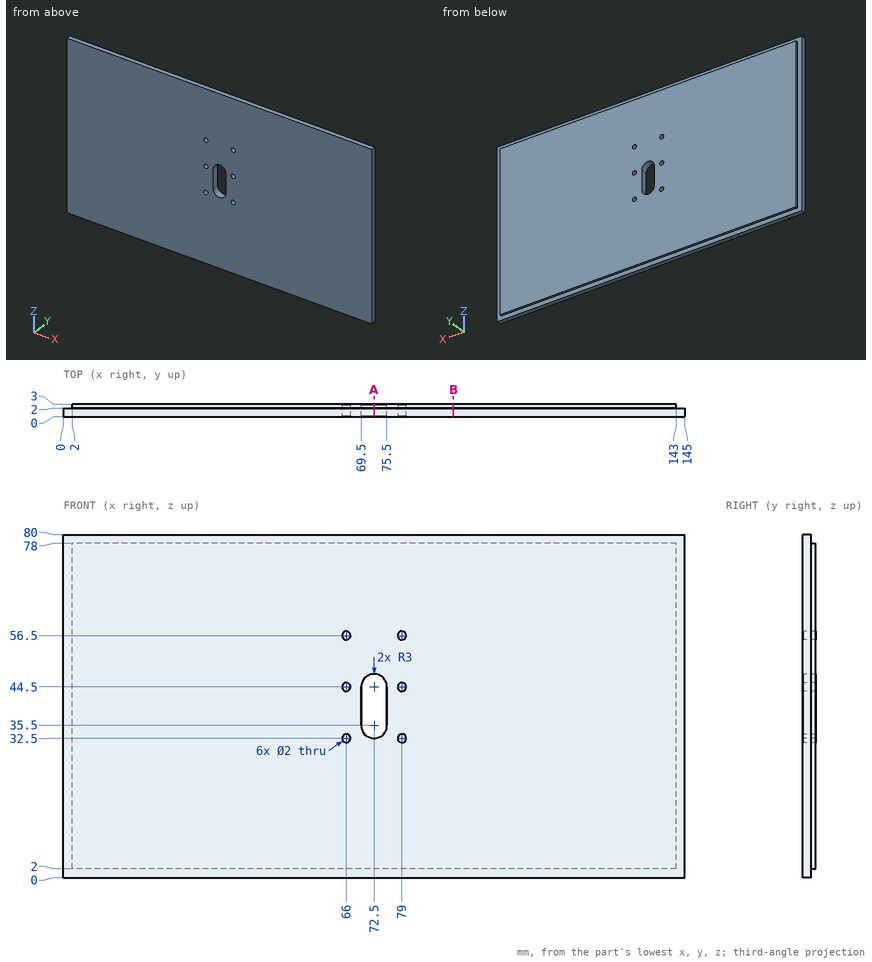
Check sheet for the drawn part. Datum: minimum x, y, z corner. Units: mm. Give positions to 0.01 mm unless a question says otherwise; leave off trailing zeros. Write each loop counter-clockwise with the first axis right and the second up, starting at its lowest first coordinate (ties: lowest second). Pieces come first, ordered by that corner, then holes. Notation, with made-up numbers: M 27.25,50.25 L 70.25,50.25 A30 ccw 70.25,83.25 Z; hole C 81.25,46.25 d8. An arc over 180 degrees is marked long. One line per question, with ' | ' between items.
1. Gauge pin test, flat ends, axial feed: pin 1 (1.2 mm diameter, centred on x = 66, z = 44.5, fed in from +Y); pin 2 (0.8 mm diameter, centred on x = 57, y = 2.5, fed in from -Z); pin 3 (0.8 mm diameter, centred on y = 2.5, z = 22, fed in from +X); pin 4 (0.8 mm diameter, centred on y = 2.5, z = 32.5, fed in from -X). Record the tip position at first contact, or that the pin passes through.
Ans:
pin 1: through | pin 2: z = 2 | pin 3: x = 143 | pin 4: x = 2
2. Scan lines: line 1 along Z through (x, y) = (79, 1.25); line 2 along Z through (x, y) = (43, 2.2); line 3 along X through (y, z) = (2.15, 6.5). Record each from-to range of solid material in increasing order. Write a range as from..to.
Ans:
line 1: 0..31.5, 33.5..43.5, 45.5..55.5, 57.5..80 | line 2: 2..78 | line 3: 2..143
3. Cross-section at A-A (x = 72.5). Enter the section's corners in (y, z).
Ans:
outline: M 0,0 L 2,0 L 2,2 L 3,2 L 3,32.5 L 0,32.5 Z; M 0,47.5 L 3,47.5 L 3,78 L 2,78 L 2,80 L 0,80 Z
4. Cross-section at B-B (x = 91). Enter the section's corners in (y, z).
Ans:
outline: M 0,0 L 2,0 L 2,2 L 3,2 L 3,78 L 2,78 L 2,80 L 0,80 Z
